Verification items for the finished model (mm, model axes). A direction names the side the tool comes from. Round coordinates to 2 decimals unless told otherwise and drop trailing zeros. Write each loop counter-clockwise with the first axis right and the second up, starting at its lowest first coordinate (ties: lowest second). Pieces come first, ordered by that corner, then holes.
from build123d import *

# Parameters (mm, degrees)
SKETCH_W          = 80
SKETCH_H          = 160
PAD_DEPTH         = 3
SKETCH001_W       = 72
SKETCH001_H       = 10
PAD001_DEPTH      = 10
SKETCH002_R       = 1.5
POCKET_DEPTH      = 76.001
POCKET_DEPTH_BACK = 4.001
FILLET_R          = 5


with BuildPart() as part:
    # Sketch → Pad (new body)
    with BuildSketch(Plane.XZ):
        Rectangle(SKETCH_W, SKETCH_H)
        Polygon((-31.5, -15), (-28, -15), (-28, -60), (28, -60), (28, -15), (31.5, -15), (31.5, 35), (28, 35), (28, 50), (-28, 50), (-28, 35), (-31.5, 35), align=None, mode=Mode.SUBTRACT)
    extrude(amount=PAD_DEPTH)

    # Sketch001 (on Face17 of Pad) → Pad001 (join)
    with BuildSketch(Plane(origin=(0, 0, 0), x_dir=(1, 0, 0), z_dir=(0, 1, 0))):
        with Locations((0, 75)):
            Rectangle(SKETCH001_W, SKETCH001_H)
        with Locations((0, -75)):
            Rectangle(SKETCH001_W, SKETCH001_H)
    extrude(amount=PAD001_DEPTH)

    # Sketch002 (on Face8 of Pad001) → Pocket (cut, two sides)
    with BuildSketch(Plane(origin=(36, 0, 0), x_dir=(0, 0, 1), z_dir=(1, 0, 0))) as pocket_sk:
        with Locations((75, -5)):
            Circle(SKETCH002_R)
        with Locations((-75, -5)):
            Circle(SKETCH002_R)
    extrude(amount=-POCKET_DEPTH, mode=Mode.SUBTRACT)
    extrude(pocket_sk.sketch, amount=POCKET_DEPTH_BACK, mode=Mode.SUBTRACT)

    # Fillet
    fillet_edges = [part.edges().sort_by_distance(p)[0] for p in [
        (0, 10, -70),
        (0, 10, 70),
    ]]
    fillet(fillet_edges, radius=FILLET_R)


solid = part.part
Q1. Sectioned sample at A-A (z = -29). Enter the section's corners in (x, y).
Recorded:
outline: (-40, -3) - (-28, -3) - (-28, 0) - (-40, 0) - close; (28, -3) - (40, -3) - (40, 0) - (28, 0) - close
Q2. Release check for a two-part mould opening along X. For faces 1 (the flat face through (-40, -1, -1)), 2 (the flat face through (30, -1, -15)), 3 (the flat face through (35, -3, 19)) record: released by +X, released by -X, zero draft, split by the parting line, or undercut.
Recorded:
face 1: released by -X
face 2: undercut
face 3: zero draft
Q3. Material ranges on line 1 along Z through (x, y) = (-8, 2); line 2 along X through (y, z) = (-0.5, 26.5); line 3 along Y through (x, z) = (9.5, -75), recorded low to high.
Recorded:
line 1: z = -80 to -70, 70 to 80
line 2: x = -40 to -31.5, 31.5 to 40
line 3: y = -3 to 3.5, 6.5 to 10
Q4. Sectioned sample at B-B (x = -14). Enter the section's corners in (y, z).
Recorded:
outline: (-3, -80) - (10, -80) - (10, -75) arc R5 ccw to (5, -70) - (0, -70) - (0, -60) - (-3, -60) - close; (-3, 50) - (0, 50) - (0, 70) - (5, 70) arc R5 ccw to (10, 75) - (10, 80) - (-3, 80) - close; hole circle Ø3 at (5, -75); hole circle Ø3 at (5, 75)
Q5. Sectioned sample at C-C (y = 8.5). Enter the section's corners in (x, z).
Recorded:
outline: (-36, -80) - (36, -80) - (36, -71.43) - (-36, -71.43) - close; (-36, 71.43) - (36, 71.43) - (36, 80) - (-36, 80) - close
Q6. Depth check by flat-ended pin: P1, Ø12, axis at x = 31.5, z = -35, coming from the +Y side; P2, Ø3.5, axis at y = 5, z = -75, coming from the -X side; P3, Ø8, axis at x = 25.5, z = -38.5, coming from the -Y side. Enter the tip coordinate at first touch or a pass-through.
Recorded:
P1: stops at y = 0
P2: stops at x = -36
P3: stops at y = -3
Q7. Sectioned sample at D-D (z = 51.5). Enter the section's corners in (x, y), plus the area to 3 significant figures.
Recorded:
outline: (-40, -3) - (40, -3) - (40, 0) - (-40, 0) - close
area: 240 mm2
Q8. Tool access check on faces 4 (the flat face through (28, -1, 42)), 5 (the cylindrical face through (1, 9, 72)), 6 (the flat face through (-36, 3.8, 76.2)). Record the directions out of +Z, -Z, +X, -X, +Y, -Y that give a thin tool (end or side, any length) a straight path to the whole face; none if there is none.
Recorded:
face 4: +Y, -Y
face 5: +X, -X, +Y
face 6: +Z, -Z, -X, +Y
